Work out the finished part from the listing and answer in its coordinate system (mm). A direction names the side the tool comes from. Give positions to 0.01 mm unless a question says otherwise; leave off trailing zeros. Order: outer loops, then holes, each group sorted by start corner. A loop starts at its lowest first (then second) coordinate and runs counter-clockwise, first axis right, second up. Notation, with made-up numbers: (20.5, 12) - (37.5, 12) arc R9 ccw to (37.5, 22) - close; hole circle Ø11 at (83.5, 82.5). An arc over 180 degrees is marked (long way). Return JSON: item names as keys, results as strings. Group by question number.
from build123d import *

# Parameters (mm, degrees)
SKETCH1_R           = 11
SKETCH1_R_2         = 5
BOSS_EXTRUDE1_DEPTH = 10
FILLET1_R           = 80
FILLET2_R           = 4


with BuildPart() as part:
    # Sketch1 → Boss-Extrude1 (new body)
    with BuildSketch(Plane.XY):
        with BuildLine():
            ThreePointArc((-55.17864045, 40), (-159.9, 0), (-55.17864045, -40))
            Line((-55.17864045, -40), (79.284471872, -40))
            ThreePointArc((79.284471872, -40), (144.9, 0), (79.284471872, 40))
            Line((79.284471872, 40), (-55.17864045, 40))
        make_face()
        with Locations((-99.9, 0)):
            Circle(SKETCH1_R, mode=Mode.SUBTRACT)
        with Locations((-39.25, 0)):
            Circle(SKETCH1_R_2, mode=Mode.SUBTRACT)
        with Locations((36.95, 0)):
            Circle(SKETCH1_R_2, mode=Mode.SUBTRACT)
        with Locations((113.15, 0)):
            Circle(SKETCH1_R_2, mode=Mode.SUBTRACT)
    extrude(amount=BOSS_EXTRUDE1_DEPTH)

    # Fillet1
    fillet1_edges = [part.edges().sort_by_distance(p)[0] for p in [
        (79.284471872, 40, 5),
        (79.284471872, -40, 5),
        (-55.17864045, -40, 5),
        (-55.17864045, 40, 5),
    ]]
    fillet(fillet1_edges, radius=FILLET1_R)

    # Fillet2
    fillet2_edges = [part.edges().sort_by_distance(p)[0] for p in [
        (18.555512755, -40, 0),
        (18.555512755, -40, 10),
        (-159.9, 0, 0),
        (-159.9, 0, 10),
        (18.555512755, 40, 0),
        (18.555512755, 40, 10),
        (144.9, 0, 0),
        (144.9, 0, 10),
        (-49.169873844, -42.910071067, 0),
        (-49.169873844, -42.910071067, 10),
        (-49.169873844, 42.910071067, 0),
        (-49.169873844, 42.910071067, 10),
        (76.213708499, -40.804040507, 0),
        (76.213708499, -40.804040507, 10),
        (76.213708499, 40.804040507, 0),
        (76.213708499, 40.804040507, 10),
    ]]
    fillet(fillet2_edges, radius=FILLET2_R)


solid = part.part
1. Each of these flat-tipped pins is pushed along its axis until it touches: pin 1 (12 mm diameter, centred on x = -21.5, y = -44, fed in from +Z); pin 2 (1 mm diameter, centred on y = 11, z = 5, fed in from +X); pin 3 (1 mm diameter, centred on x = -0.5, z = 5.5, fed in from +Y); pin 4 (6 mm diameter, centred on x = 36.95, y = 0, fed in from -Z). Where does it stop, or does it pass through?
2. Consider probe 1 along Y at (x, z) = (-99.9, 6); probe 2 along Y at (x, z) = (112.5, 6.5); probe 3 along Y at (x, z) = (12, 3.75). Determine where each line is inside the solid, lowest interval first. Write a range as from..to.
3. Determine the mould class of faces 1 (the cylindrical face through (-44.245, 0.22, 4.93)), 2 (the flat face through (-10, 1, 0)), 3 (the cylindrical face through (144.885, -1.168, 4.986)) for opening direction Y: released by +Y, released by -Y, zero draft, split by the parting line, or undercut.
4. The part is cut by section B-B (x = -18). Give the vertices of the cut face in (y, z), and give its area (3 significant figures).
5. A tool of negligible diameter and unlimited length cuts with its end or side. For faces 4 (the cylindrical face through (-49.46, -42.99, 5.01)), 5 (the cylindrical face through (-159.874, 1.774, 4.986)), 6 (the cylindrical face through (-49.46, 42.99, 5.01)), from which of +Z, -Z, +X, -X, +Y, -Y can it reach the whole face along a straight path? Write none if from no direction.
6. The part is cut by section A-A (x = 36.95). Give the vertices of the cut face in (y, z).
Answers:
{
 "1": {"pin 1": "stops at z = 9.46", "pin 2": "stops at x = 143.66", "pin 3": "stops at y = 40", "pin 4": "passes through"},
 "2": {"probe 1": "y = -60..-11, 11..60", "probe 2": "y = -43.17..-4.96, 4.96..43.17", "probe 3": "y = -39.99..39.99"},
 "3": {"face 1": "undercut", "face 2": "zero draft", "face 3": "split by the parting line"},
 "4": {"outline": "(-40, 4) arc R4 ccw to (-36, 0) - (36, 0) arc R4 ccw to (40, 4) - (40, 6) arc R4 ccw to (36, 10) - (-36, 10) arc R4 ccw to (-40, 6) - close", "area": "786 mm^2"},
 "5": {"face 4": "+Z, -Z, -Y", "face 5": "+Z, -Z", "face 6": "+Z, -Z, +Y"},
 "6": {"outline": "(-40, 4) arc R4 ccw to (-36, 0) - (-5, 0) - (-5, 10) - (-36, 10) arc R4 ccw to (-40, 6) - close; (5, 0) - (36, 0) arc R4 ccw to (40, 4) - (40, 6) arc R4 ccw to (36, 10) - (5, 10) - close"}
}
